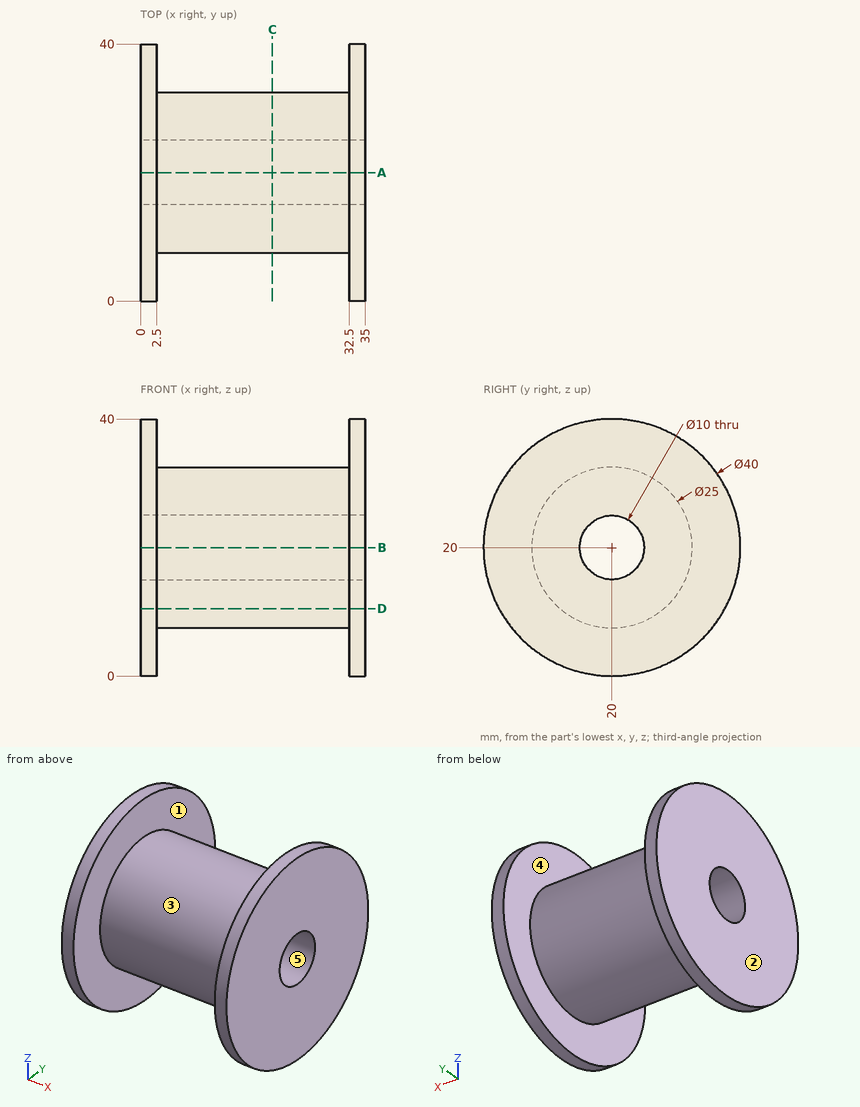
Geometry: see drawing. Coordinates: mm, zero at the bounding-box minimum. A direction names the side the tool comes from. Give positions to 0.01 mm unless a question says otherwise; leave off trailing zeros. Write each loop counter-clockwise with the first axis right and the second up, starting at its lowest first coordinate (ties: lowest second). Pieces come first, ordered by that corner, then holes. Notation, with made-up numbers: (56, -11.75) - (87, -11.75) arc R25 ccw to (87, 14.25) - close; hole circle Ø1 at (58, -1). An arc over 180 degrees is marked (long way). Return JSON: item names as keys, results as strings. Group by question number.
1) Section D-D on z = 10.5. Return the cut outline in (x, y), plus the area to 3 significant figures.
2) Section C-C on x = 20.5. Return the cut outline in (y, z).
3) Section A-A on y = 20. Return the cut outline in (x, z).
4) First-contact query: P1, Ø10, axis at x = 10.5, y = 33.5, coming from the -Z side; P2, Ø4, axis at x = 15.5, z = 17.5, coming from the +Y side; P3, Ø12, axis at y = 16, z = 19, coming from the -X side; P4, Ø1.5, axis at x = 16, z = 12, coming from the +Y side. Flat tips, straight axial feed; report the tip coordinate or a pass-through.
5) Set-up query: the marked faces 1 and 2. Return all of +Z, -Z, +X, -X, +Y, -Y with unobstructed straight access to the full face (end or side cutting, diameter ignored); none if empty.
6) Line query: line 1 (X direction, y = 10, z = 30); line 2 (Y direction, x = 17, z = 20); line 3 (Z direction, x = 12, y = 18.5). Output: solid intervals per line, ascending.
7) Mould query, pull axis Y, two halves, no side actions, for the marked faces 3, 4 and 5. Classes: released by +Y, released by -Y, zero draft, split by the parting line, or undercut.
Filled in:
{
 "1": {"outline": "(0, 2.4) - (2.5, 2.4) - (2.5, 11.88) - (32.5, 11.88) - (32.5, 2.4) - (35, 2.4) - (35, 37.6) - (32.5, 37.6) - (32.5, 28.12) - (2.5, 28.12) - (2.5, 37.6) - (0, 37.6) - close", "area": "663 mm^2"},
 "2": {"outline": "circle Ø25 at (20, 20); hole circle Ø10 at (20, 20)"},
 "3": {"outline": "(0, 0) - (2.5, 0) - (2.5, 7.5) - (32.5, 7.5) - (32.5, 0) - (35, 0) - (35, 15) - (0, 15) - close; (0, 25) - (35, 25) - (35, 40) - (32.5, 40) - (32.5, 32.5) - (2.5, 32.5) - (2.5, 40) - (0, 40) - close"},
 "4": {"P1": "stops at z = 10.83", "P2": "stops at y = 32.49", "P3": "stops at x = 0", "P4": "stops at y = 30.18"},
 "5": {"face 1": "none", "face 2": "+Z, -Z, -X, +Y, -Y"},
 "6": {"line 1": "x = 0 to 2.5, 32.5 to 35", "line 2": "y = 7.5 to 15, 25 to 32.5", "line 3": "z = 7.59 to 15.23, 24.77 to 32.41"},
 "7": {"face 3": "split by the parting line", "face 4": "zero draft", "face 5": "undercut"}
}
